from build123d import *

# Parameters (mm, degrees)
SKETCH2_R          = 15.716456716
CUT_EXTRUDE2_DEPTH = 12
SKETCH3_R          = 15.643449511
CUT_EXTRUDE3_DEPTH = 5
FILLET1_R          = 2


with BuildPart() as part:
    # Sketch1 → Revolve1 (revolve)
    with BuildSketch(Plane.XY, mode=Mode.PRIVATE) as revolve1_sk:
        Polygon((0, 4.25), (28.652506034, 4.25), (28.652506034, 8.798665847), (24.864443275, 8.798665847), (24.864443275, 11), (14.352506034, 11), (14.352506034, 7.20220566), (11.591810477, 7.20220566), (11.591810477, 10), (8, 10), (8, 6.5), (0, 6.5), align=None)
    revolve(revolve1_sk.sketch.rotate(Axis((0, 0, 0), (1, 0, 0)), 90), axis=Axis((0, 0, 0), (1, 0, 0)))

    # Sketch2 → Cut-Extrude2 (cut)
    with BuildSketch(Plane(origin=(24.864443275, 0, 0), x_dir=(0, 0, -1), z_dir=(1, 0, 0))):
        Circle(SKETCH2_R)
        Polygon((0, 10.392304845), (-9, 5.196152423), (-9, -5.196152423), (0, -10.392304845), (9, -5.196152423), (9, 5.196152423), align=None, mode=Mode.SUBTRACT)
    extrude(amount=-CUT_EXTRUDE2_DEPTH, mode=Mode.SUBTRACT)

    # Sketch3 → Cut-Extrude3 (cut)
    with BuildSketch(Plane.ZY.offset(-8)):
        Circle(SKETCH3_R)
        Polygon((0, 9.237604307), (-8, 4.618802154), (-8, -4.618802154), (0, -9.237604307), (8, -4.618802154), (8, 4.618802154), align=None, mode=Mode.SUBTRACT)
    extrude(amount=-CUT_EXTRUDE3_DEPTH, mode=Mode.SUBTRACT)

    # Fillet1
    fillet1_edges = [part.edges().sort_by_distance(p)[0] for p in [
        (28.652506034, 0, -8.798665847),
    ]]
    fillet(fillet1_edges, radius=FILLET1_R)


solid = part.part
For this review, take the finished solid that the model builds, in its own axes (mm). A direction names the side the tool comes from. Round coordinates to 2 decimals unless told otherwise and drop trailing zeros. Loops run counter-clockwise (first coordinate to the right, second up) from the corner with the lowest first, then second, coordinate; pieces in that order, holes last. Notation, with made-up numbers: (39.25, 53.25) - (77.25, 53.25) arc R33 cw to (77.25, 81.25) - close; hole circle Ø11 at (3.25, -23). An arc over 180 degrees is marked (long way). Use one line per item in the form item = value.
1) Mouldability with a two-part tool opening along X and no side actions: class faces 1 (the face through (14.353, 5, -6)), 2 (the face through (10, 0, 8)), 3 (the face through (24.864, 9, 0)), 4 (the face through (8, 3, -6)) as pulls with the +X half, pulls with the -X half, needs draft (parallel to the pull), parting line crosses it, or undercut.
Solutions:
face_1 = undercut
face_2 = needs draft
face_3 = pulls with the +X half
face_4 = pulls with the -X half
2) Wall thickness on probe 1 along Y at (x, z) = (24.5, -1.75); probe 2 along X at (y, z) = (3.5, -6.5); probe 3 along Y at (x, z) = (2.75, -2): over which ranges is each line inside the solid? List them lowest first.
Solutions:
probe_1 = -9.38 to -3.87, 3.87 to 9.38
probe_2 = 8 to 11.59, 14.35 to 28.57
probe_3 = -6.18 to -3.75, 3.75 to 6.18
3) We need section A-A on y = 0. Write out the cut boundary in (x, z), then the cut area to 3 significant figures.
Solutions:
outline = (0, -6.5) - (8, -6.5) - (8, -8) - (11.59, -8) - (11.59, -7.2) - (14.35, -7.2) - (14.35, -9) - (24.86, -9) - (24.86, -8.8) - (26.65, -8.8) arc R2 ccw to (28.65, -6.8) - (28.65, -4.25) - (0, -4.25) - close; (0, 4.25) - (28.65, 4.25) - (28.65, 6.8) arc R2 ccw to (26.65, 8.8) - (24.86, 8.8) - (24.86, 9) - (14.35, 9) - (14.35, 7.2) - (11.59, 7.2) - (11.59, 8) - (8, 8) - (8, 6.5) - (0, 6.5) - close
area = 212 mm2
4) We need section B-B on x = 9. Write out the cut boundary in (y, z).
Solutions:
outline = (-9.24, 0) - (-4.62, -8) - (4.62, -8) - (9.24, 0) - (4.62, 8) - (-4.62, 8) - close; hole circle Ø8.5 at (0, 0)
5) We need section D-D on x = 3. Write out the cut boundary in (y, z), then the cut area to 3 significant figures.
Solutions:
outline = circle Ø13 at (0, 0); hole circle Ø8.5 at (0, 0)
area = 76.0 mm2
6) We need section C-C on x = 22.25. Write out the cut boundary in (y, z).
Solutions:
outline = (-10.39, 0) - (-5.2, -9) - (5.2, -9) - (10.39, 0) - (5.2, 9) - (-5.2, 9) - close; hole circle Ø8.5 at (0, 0)
7) Clearance check with flat-ended pins moving along their axes: P1, Ø1, axis at x = 10.5, z = 5.5, coming from the +Y side; P2, Ø3, axis at x = 10, y = 1.5, coming from the -Z side; P3, Ø1.8, axis at x = 10, y = -2, coming from the +Z side. State where each tip first meets the part, or that it passes through.
Solutions:
P1 = 6.35
P2 = -8
P3 = 8
8) Tool access review of faces 5 (the face through (10, 0, -8)), 6 (the face through (25.75, 8.59, -1.91)), 7 (the face through (3.944, 3.955, -5.158)): name each direction out of +Z, -Z, +X, -X, +Y, -Y from which nothing blocks a thin tool from reaching the whole face with its end or side.
Solutions:
face_5 = -Z, -X, +Y, -Y
face_6 = +X
face_7 = -X
